Read the model definition and answer for the solid it produces. Units are mm, in the model's axes. Face numbers are marked on the shaded views. A direction names the side the tool comes from. Coordinates: 2 decimals unless noted, no trailing zeros. Loops run counter-clockwise (first coordinate to the right, second up) from the corner with the lowest first, then second, coordinate; pieces in that order, holes last. Notation, with made-up numbers: (38, 17.5) - (67, 17.5) arc R23 cw to (67, 46.5) - close; hole circle Ø1 at (31.5, 76.5). An arc over 180 degrees is marked (long way). One line per item, written item: value. Start each with the question number.
Autodesk Inventor part; units mm, degrees
ref_plane "YZ Plane" through (0, 0, 0) normal (1, 0, 0) x (0, 1, 0)
ref_plane "XZ Plane" through (0, 0, 0) normal (0, 1, 0) x (-1, 0, 0)
ref_plane "XY Plane" through (0, 0, 0) normal (0, 0, 1) x (1, 0, 0)
sketch "Sketch1" plane through (0, 0, 0) normal (0, 0, 1) x (1, 0, 0)
  circle A0 centre (0, 0) radius 100
  dimension "d0" = 200
extrude "Extrusion1" add sketch "Sketch1" along normal blind 250
sketch "Sketch2" plane through (0, 0, 250) normal (0, 0, 1) x (1, 0, 0)
  circle A0 centre (0, 0) radius 100
  line L0 (-100, 50) -> (-100, -50) construction
  dimension "d3" = 100
  dimension "d4" = 50
ref_plane "Work Plane1" through (0, 0, 250) normal (0, -1, 0) x (1, 0, 0)
sketch "Sketch3" plane through (0, 0, 250) normal (0, -1, 0) x (1, 0, 0)
  line L0 (100, 0) -> (-100, 0)
  line L1 (100, 0) -> (0, 0)
  line L2 (0, 0) -> (0, -150)
  line L3 (0, -150) -> (100, -150)
  line L4 (100, -150) -> (100, 0)
  point P0 (0, -250)
  point P1 (0, 0)
  dimension "d6" = 150
  dimension "d17" = 100
extrude "Extrusion2" cut sketch "Sketch3" along normal through all both and the other way through all
sketch "Sketch4" plane through (0, -50, 125) normal (1, 0, 0) x (0, 0, -1)
  circle A0 centre (-75, 50) radius 5
  line L0 (-125, -50) -> (-125, 150)
  point P0 (125, 50)
  dimension "d9" = 10
  dimension "d18" = 50
hole "Hole1" at (0, 0, 200) direction (-1, 0, 0) diameter 10 end through all
equation "\"d18\" = 0.5 * d3"
properties part number "link1"
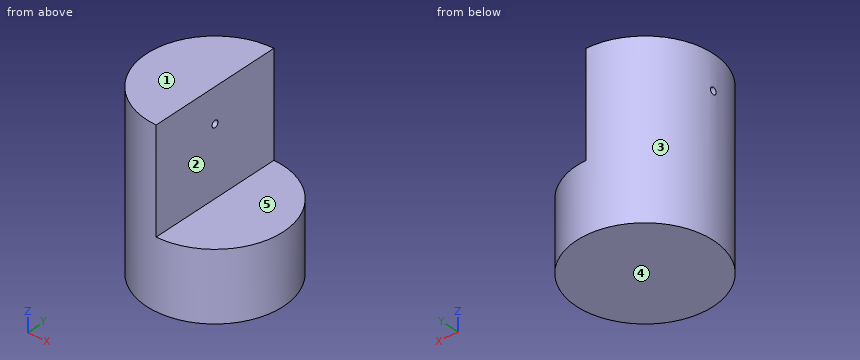
1) For the marked faces 4 and 5, determine the directions among +Z, -Z, +X, -X, +Y, -Y from which every point of the face is accessible in a straight line to the end or side of a thin tool.
2) Determine the mould class of the marked faces 1, 2 and 3 for opening direction X: released by +X, released by -X, zero draft, split by the parting line, or undercut.
3) Section C-C, the plane x = -36 is taken. Determine the outline of the cut face in (y, z), and give its area (3 significant figures).
4) Section D-D, the plane y = 34 is taken. Determine the outline of the cut face in (x, z), and give its area (3 significant figures).
5) Straight lines are drawn through the part: L1, parallel to Z at x = -73, y = 0; L2, parallel to Z at x = 20, y = -4.5; L3, parallel to X at y = -2.5, z = 67.5. For each, find the intervals that lie inside material, in ascending order.
6) Section A-A, the plane y = 0 is taken. Determine the outline of the cut face in (x, z).
7) Section B-B, the plane z = 200 is taken. Determine the outline of the cut face in (x, y).
8) Flat-ended cylindrical pins translate along their axes: P1, Ø1.5, axis at x = 52, y = -53.5, coming from the -Z side; P2, Ø5, axis at y = 48, z = 72.5, coming from the +X side; P3, Ø12, axis at x = 69, y = -73, coming from the +Z side; P4, Ø8, axis at x = -68.5, z = 190.5, coming from the -Y side. Find the tip coordinate at first contact, or state that the pin passes through.
Answer below:
1. face 4: -Z, +X, -X, +Y, -Y
1. face 5: +Z, +X, +Y, -Y
2. face 1: zero draft
2. face 2: released by +X
2. face 3: split by the parting line
3. outline: (-93.3, 0) - (93.3, 0) - (93.3, 250) - (-93.3, 250) - close; hole circle Ø10 at (0, 200)
3. area: 46,600 mm2
4. outline: (-94.04, 0) - (94.04, 0) - (94.04, 100) - (0, 100) - (0, 250) - (-94.04, 250) - close
4. area: 32,900 mm2
5. L1: 0 to 195, 205 to 250
5. L2: 0 to 100
5. L3: -99.97 to 99.97
6. outline: (-100, 0) - (100, 0) - (100, 100) - (0, 100) - (0, 195) - (-100, 195) - close; (-100, 205) - (0, 205) - (0, 250) - (-100, 250) - close
7. outline: (-99.87, -5) arc R100 ccw to (0, -100) - (0, -5) - close; (-99.87, 5) - (0, 5) - (0, 100) arc R100 ccw to start
8. P1: z = 0
8. P2: x = 89.05
8. P3: z = 100
8. P4: y = -76.42
